Autodesk Inventor part; units mm, degrees
ref_plane "YZ Plane" through (0, 0, 0) normal (1, 0, 0) x (0, 1, 0)
ref_plane "XZ Plane" through (0, 0, 0) normal (0, 1, 0) x (-1, 0, 0)
ref_plane "XY Plane" through (0, 0, 0) normal (0, 0, 1) x (1, 0, 0)
sketch "スケッチ1" plane through (0, 0, 0) normal (0, 0, 1) x (1, 0, 0)
  arc A0 (0, 53.5) -> (-53.5, 0) centre (0, 0) ccw
  line L0 (-60.5, 0) -> (-60.5, 60.5)
  line L1 (-60.5, 60.5) -> (0, 60.5)
  line L2 (0, 60.5) -> (0, -99.4363)
  line L3 (-60.5, 0) -> (-60.5, -25)
  line L4 (-60.5, -25) -> (-53.5, -25)
  line L5 (-53.5, -25) -> (-53.5, 0)
  dimension "d0" = 107
  dimension "d3" = 25
extrude "押し出し1" add sketch "スケッチ1" along normal blind 85
sketch "スケッチ2" plane through (-60.5, 60.5, 0) normal (0, 1, 0) x (1, 0, 0)
  line L0 (60.5, -85) -> (7, -85)
  line L1 (60.5, -85) -> (60.5, -42.5)
  line L2 (60.5, 0) -> (60.5, -85)
  line L3 (60.5, -42.5) -> (40.18, -42.5)
  line L4 (40.18, -42.5) -> (40.18, -5.67)
  line L5 (40.18, -42.5) -> (40.18, -79.33)
  circle A0 centre (40.18, -5.67) radius 1.6
  circle A1 centre (40.18, -79.33) radius 1.6
  line L6 (60.5, -42.5) -> (-11.6627, -42.5)
  line L7 (-11.6627, -42.5) -> (-11.6627, -99.0684)
  line L8 (-11.6627, -99.0684) -> (60.5, -99.0684)
  line L9 (60.5, -99.0684) -> (60.5, -42.5)
  dimension "d8" = 20.32
  dimension "d9" = 36.83
  dimension "d10" = 36.83
  dimension "d11" = 3.2
  dimension "d12" = 3.2
extrude "押し出し2" cut sketch "スケッチ2" against normal through all contours A1 | A0
ref_plane "作業平面1" through (-60.5, 42.25, 0) normal (0, 1, 0) x (1, 0, 0)
sketch "スケッチ3" plane through (-60.5, 42.25, 0) normal (0, 1, 0) x (1, 0, 0)
  circle A0 centre (40.18, -5.67) radius 1.6
  line L0 (43.53, -5.67) -> (41.855, -8.5712)
  line L1 (41.855, -8.5712) -> (38.505, -8.5712)
  line L2 (38.505, -8.5712) -> (36.83, -5.67)
  line L3 (36.83, -5.67) -> (38.505, -2.7688)
  line L4 (38.505, -2.7688) -> (41.855, -2.7688)
  line L5 (41.855, -2.7688) -> (43.53, -5.67)
  point P0 (60.5, 0)
  dimension "d16" = 6.7
extrude "押し出し3" cut sketch "スケッチ3" along normal blind 11
extrude "押し出し4" cut sketch "スケッチ2" against normal through all contours L9 L8 L7 L6 L3 L1
mirror "ミラー1" about plane through (-72.1627, 60.5, 42.5) normal (0, 0, 1)
sketch "スケッチ4" plane through (-60.5, -25, 0) normal (-1, 0, 0) x (0, 0, 1)
  line L0 (85, 78.5) -> (0, 78.5)
  line L1 (0, 78.5) -> (85, 78.5)
  line L2 (85, 25) -> (0, 25)
  line L3 (0, 25) -> (85, 25)
  line L4 (0, 25) -> (0, 12.5)
  line L5 (0, 85.5) -> (0, 0)
  line L6 (0, 12.5) -> (85, 12.5)
  line L7 (85, 0) -> (85, 25)
  circle A0 centre (20, 12.5) radius 2.1
  line L8 (85, 12.5) -> (65, 12.5)
  circle A1 centre (65, 12.5) radius 2.1
  dimension "d21" = 12.5
  dimension "d22" = 4.2
  dimension "d23" = 20
  dimension "d24" = 20
  dimension "d25" = 4.2
extrude "押し出し5" cut sketch "スケッチ4" against normal blind 10 contours A1 L6 | L6 A1 | A0 L6 | L6 A0
fillet "フィレット1" radius 5 1 edges at (-60.5, 60.5, 42.5)
mirror "ミラー2" about plane through (0, 53.5, 0) normal (1, 0, 0)
properties part number "mainIMU"
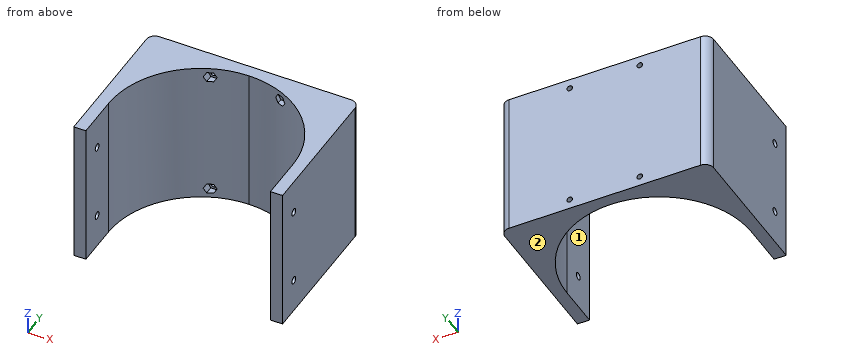
Here's how the part is built. I have some questions about the finished solid (model axes, mm). Face numbers are marked on the shaded views. A direction names the side the tool comes from. Coordinates: 2 decimals unless noted, no trailing zeros. Write each loop counter-clockwise with the first axis right and the second up, starting at its lowest first coordinate (ties: lowest second). Pieces come first, ordered by that corner, then holes. Notation, with made-up numbers: (15, 22.5) - (46, 22.5) arc R21 cw to (46, 52.5) - close; hole circle Ø9 at (-35, 80). An arc over 180 degrees is marked (long way). One line per item, written item: value.
1) Suppose I cut it at A-A on y = -12.5. Write out the boundary of the cut face in (x, z).
Model answer:
outline: (-60.5, 0) - (-53.5, 0) - (-53.5, 17.9) - (-60.5, 17.9) - close; (-60.5, 22.1) - (-53.5, 22.1) - (-53.5, 62.9) - (-60.5, 62.9) - close; (-60.5, 67.1) - (-53.5, 67.1) - (-53.5, 85) - (-60.5, 85) - close; (53.5, 0) - (60.5, 0) - (60.5, 17.9) - (53.5, 17.9) - close; (53.5, 22.1) - (60.5, 22.1) - (60.5, 62.9) - (53.5, 62.9) - close; (53.5, 67.1) - (60.5, 67.1) - (60.5, 85) - (53.5, 85) - close
2) Suppose I cut it at D-D on y = 22. Write out the boundary of the cut face in (x, z).
Model answer:
outline: (-60.5, 0) - (-48.77, 0) - (-48.77, 85) - (-60.5, 85) - close; (48.77, 0) - (60.5, 0) - (60.5, 85) - (48.77, 85) - close
3) Suppose I cut it at B-B on z = 65. Write out the boundary of the cut face in (x, y).
Model answer:
outline: (-60.5, -25) - (-53.5, -25) - (-53.5, -14.6) - (-60.5, -14.6) - close; (-60.5, -10.4) - (-53.5, -10.4) - (-53.5, 0) arc R53.5 cw to (53.5, 0) - (53.5, -10.4) - (60.5, -10.4) - (60.5, 55.5) arc R5 ccw to (55.5, 60.5) - (-55.5, 60.5) arc R5 ccw to (-60.5, 55.5) - close; (53.5, -25) - (60.5, -25) - (60.5, -14.6) - (53.5, -14.6) - close
4) Suppose I cut it at C-C on x = -20.32. Write out the boundary of the cut face in (y, z).
Model answer:
outline: (49.49, 0) - (60.5, 0) - (60.5, 4.07) - (53.25, 4.07) - (53.25, 2.77) - (49.49, 2.77) - close; (49.49, 8.57) - (53.25, 8.57) - (53.25, 7.27) - (60.5, 7.27) - (60.5, 77.73) - (53.25, 77.73) - (53.25, 76.43) - (49.49, 76.43) - close; (49.49, 82.23) - (53.25, 82.23) - (53.25, 80.93) - (60.5, 80.93) - (60.5, 85) - (49.49, 85) - close
5) I need wall thicknesses on line 1 along Z through (x, y) = (56.5, -12.5); line 2 along Z through (x, y) = (20, 55); line 3 along X through (y, z) = (-15, 34.5). Which ranges of each line are inside material? Lowest first, please.
Model answer:
line 1: z = 0 to 17.9, 22.1 to 62.9, 67.1 to 85
line 2: z = 0 to 4.1, 7.24 to 77.76, 80.9 to 85
line 3: x = -60.5 to -53.5, 53.5 to 60.5
6) On a 3-axis mill with a long thin cutter (end or side, diameter ignored), from which of +Z, -Z, +X, -X, +Y, -Y can I reach the whole of each face in a straight line? I mean the marked faces 1 and 2. Say none if no direction works.
Model answer:
face 1: +Z, -Z, -Y
face 2: -Z, +X, -X, +Y, -Y
7) I'm going to push flat-ended pins straight in: P1, Ø4.5, axis at x = -21.5, z = 6, coming from the -Y side; P2, Ø4, axis at x = 20.32, z = 5.67, coming from the -Y side; P3, Ø3, axis at x = -2.5, z = 69.5, coming from the -Y side. Where does each tip first touch, or does it pass through?
Model answer:
P1: stops at y = 47.94
P2: stops at y = 53.25
P3: stops at y = 53.35
